Verification items for the finished model (mm, model axes). Face numbers are marked on the shaded views. A direction names the side the tool comes from. Coordinates: 2 decimals unless noted, no trailing zeros. Loops run counter-clockwise (first coordinate to the right, second up) from the corner with the lowest first, then second, coordinate; pieces in that order, holes last. Notation, with made-up numbers: (40.25, 14.25) - (48.25, 14.25) arc R28 ccw to (48.25, 48.25) - close; hole circle Ø9 at (-39.5, 78). An arc over 180 degrees is marked (long way). One line per item, written item: value. Start each with the question number.
(1) Draft check along X on the marked faces 1, 2 and 3. Enter one of: +X half, -X half, draft (parallel to the pull), parting line (faces both ways), or undercut.
(2) Section check D-D (y = 2.5). Record the boundary of the cut face in (x, z).
(3) Gauge pin test, flat ends, axial feed: P1, Ø3, axis at y = 3, z = -1.5, coming from the +X side; P2, Ø1.5, axis at x = 1, y = 3, coming from the +Z side; P3, Ø2.5, axis at x = 0, z = 0, coming from the +Y side. Record the tip position at first contact, or that the pin passes through.
(4) Section check A-A (y = 4.5). Record the boundary of the cut face in (x, z).
(5) Set-up check for the marked faces 4 and 5: record each of +Z, -Z, +X, -X, +Y, -Y from which the full face is reachable in a straight line by a thin tool's end or side.
(6) Section check B-B (x = 1.8). Count the separate pieces of the cut face and the enclosed holes in it, plus the area to 3 significant figures.
(7) Thickness scan on probe 1 along Y at (x, z) = (-0.75, 2.1); probe 2 along Y at (x, z) = (-1.3, 1.8); probe 3 along X at (y, z) = (3, -1.1). Record the ranges inside material, lowest first. Write a range as [from, to].
```python
from build123d import *

# Parameters (mm, degrees)
FILLET1_R = 0.635


with BuildPart() as part:
    # Sketch1 → Revolve1 (revolve)
    with BuildSketch(Plane.XY):
        with BuildLine():
            Line((-1.397, 7.874), (-2.413, 7.874))
            Line((-2.413, 7.874), (-1.524, 6.428919943))
            ThreePointArc((-1.524, 6.428919943), (-2.921, 3.937), (-1.524, 1.445080057))
            Line((-1.524, 1.445080057), (-2.413, 0))
            Line((-2.413, 0), (-1.397, 0))
            Line((-1.397, 0), (-1.397, 7.874))
        make_face()
    revolve(axis=Axis((0, 0, 0), (0, 1, 0)))

    # Fillet1
    fillet1_edges = [part.edges().sort_by_distance(p)[0] for p in [
        (1.524, 1.445080057, 0),
        (1.524, 6.428919943, 0),
    ]]
    fillet(fillet1_edges, radius=FILLET1_R)


solid = part.part
```
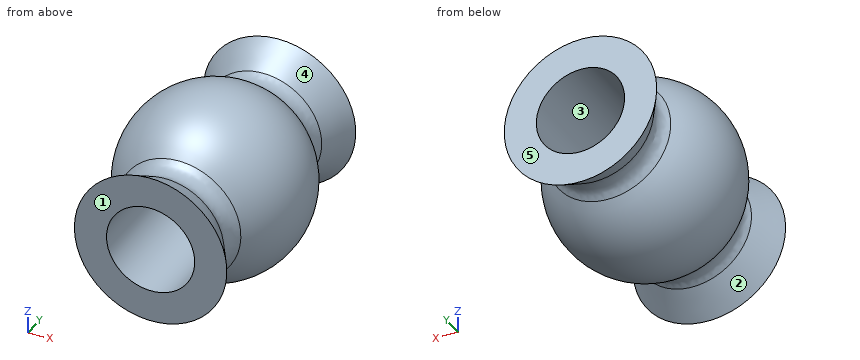
Responses:
1. face 1: draft
1. face 2: parting line
1. face 3: undercut
2. outline: circle Ø5.09 at (0, 0); hole circle Ø2.79 at (0, 0)
3. P1: stops at x = 2.91
3. P2: stops at z = 2.85
3. P3: passes through
4. outline: circle Ø5.73 at (0, 0); hole circle Ø2.79 at (0, 0)
5. face 4: none
5. face 5: +Z, -Z, +X, -X, +Y
6. separate pieces: 3
6. enclosed holes: 0
6. area: 20.9 mm²
7. probe 1: y = [0, 0.3], [2.05, 5.82], [7.58, 7.87]
7. probe 2: y = [0, 0.31], [2.04, 5.83], [7.56, 7.87]
7. probe 3: x = [-2.54, -0.86], [0.86, 2.54]
